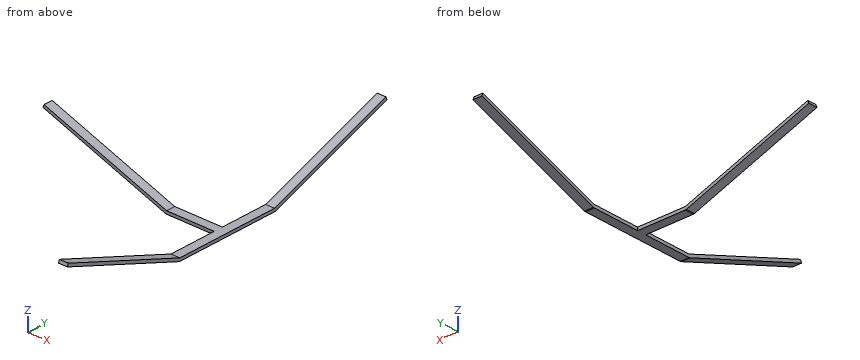
```python
from build123d import *

# Parameters (mm, degrees)
BOSS_EXTRUDE1_DEPTH  = 350
SKETCH2_W            = 150
SKETCH2_H            = 350
BOSS_EXTRUDE2_DEPTH  = 350
BOSS_EXTRUDE3_DEPTH  = 350
BOSS_EXTRUDE4_DEPTH  = 350
SKETCH6_W            = 438.570660024
SKETCH6_H            = 30
CUT_EXTRUDE1_DEPTH   = 10
CUT_EXTRUDE2_DEPTH   = 10
SKETCH8_W            = 30
SKETCH8_H            = 438.570660025
CUT_EXTRUDE3_DEPTH   = 10
SKETCH9_W            = 30
SKETCH9_H            = 438.570660025
CUT_EXTRUDE4_DEPTH   = 10
SKETCH12_W           = 438.570660024
SKETCH12_H           = 30
BOSS_EXTRUDE5_DEPTH  = 10
BOSS_EXTRUDE6_DEPTH  = 10
SKETCH14_W           = 30
SKETCH14_H           = 438.570660025
BOSS_EXTRUDE7_DEPTH  = 10
SKETCH15_W           = 30
SKETCH15_H           = 438.570660025
BOSS_EXTRUDE8_DEPTH  = 10
BOSS_EXTRUDE10_DEPTH = 30
BOSS_EXTRUDE11_DEPTH = 30
BOSS_EXTRUDE12_DEPTH = 30
SKETCH20_W           = 438.570660024
SKETCH20_H           = 160
CUT_EXTRUDE5_DEPTH   = 1000
SKETCH21_W           = 438.570660024
SKETCH21_H           = 160
CUT_EXTRUDE6_DEPTH   = 1000
SKETCH22_W           = 160
SKETCH22_H           = 160
CUT_EXTRUDE7_DEPTH   = 1000
SKETCH23_W           = 160
SKETCH23_H           = 160
CUT_EXTRUDE8_DEPTH   = 1000
SKETCH24_W           = 160
SKETCH24_H           = 438.570660025
CUT_EXTRUDE9_DEPTH   = 1000
SKETCH25_W           = 160
SKETCH25_H           = 438.570660025
CUT_EXTRUDE10_DEPTH  = 1000
SKETCH26_W           = 160
SKETCH26_H           = 350
CUT_EXTRUDE11_DEPTH  = 1000
SKETCH27_W           = 160
SKETCH27_H           = 438.570660025
CUT_EXTRUDE12_DEPTH  = 1000
SKETCH28_W           = 160
SKETCH28_H           = 438.570660025
CUT_EXTRUDE13_DEPTH  = 1000
CUT_EXTRUDE14_DEPTH  = 1000
CUT_EXTRUDE15_DEPTH  = 1000


with BuildPart() as part:
    # Sketch1 → Boss-Extrude1 (new body)
    with BuildSketch(Plane(origin=(0, 0, 0), x_dir=(1, 0, 0), z_dir=(0, 1, 0))):
        Polygon((0, 0), (412.121612918, 0), (412.121612918, 150), align=None)
    extrude(amount=BOSS_EXTRUDE1_DEPTH)

    # Sketch2 → Boss-Extrude2 (add)
    with BuildSketch(Plane(origin=(412.121612918, 0, 0), x_dir=(0, 0, -1), z_dir=(1, 0, 0))):
        with Locations((75, 175)):
            Rectangle(SKETCH2_W, SKETCH2_H)
    extrude(amount=BOSS_EXTRUDE2_DEPTH)

    # Sketch4 → Boss-Extrude3 (add)
    with BuildSketch(Plane(origin=(762.121612918, 0, 0), x_dir=(0, 0, -1), z_dir=(1, 0, 0))):
        Polygon((0, 762.121612918), (150, 350), (0, 350), align=None)
    extrude(amount=-BOSS_EXTRUDE3_DEPTH)

    # Sketch5 → Boss-Extrude4 (add)
    with BuildSketch(Plane(origin=(762.121612918, 0, 0), x_dir=(0, 0, -1), z_dir=(1, 0, 0))):
        Polygon((0, 0), (0, -412.121612918), (150, 0), align=None)
    extrude(amount=-BOSS_EXTRUDE4_DEPTH)

    # Sketch6 → Cut-Extrude1 (cut)
    with BuildSketch(Plane(origin=(0, 0, 0), x_dir=(-0.9396926207859104, 0, 0.34202014332566316), z_dir=(-0.34202014332566316, 0, -0.9396926207859104))):
        with Locations((-219.285330012, 175)):
            Rectangle(SKETCH6_W, SKETCH6_H)
    extrude(amount=-CUT_EXTRUDE1_DEPTH, mode=Mode.SUBTRACT)

    # Sketch7 → Cut-Extrude2 (cut)
    with BuildSketch(Plane(origin=(0, 0, -150), x_dir=(-1, 0, 0), z_dir=(0, 0, -1))):
        Polygon((-412.121612918, 190), (-572.121612918, 190), (-572.121612918, 350), (-602.121612918, 350), (-602.121612918, 190), (-602.121612918, 164.900861359), (-602.121612918, 160), (-602.121612918, 0), (-572.121612918, 0), (-572.121612918, 160), (-412.121612918, 160), align=None)
    extrude(amount=-CUT_EXTRUDE2_DEPTH, mode=Mode.SUBTRACT)

    # Sketch8 → Cut-Extrude3 (cut)
    with BuildSketch(Plane(origin=(0, -48.209070726, -132.453333234), x_dir=(-1, 0, 0), z_dir=(0, -0.34202014332566283, -0.9396926207859106))):
        with Locations((-587.121612918, -167.982308514)):
            Rectangle(SKETCH8_W, SKETCH8_H)
    extrude(amount=-CUT_EXTRUDE3_DEPTH, mode=Mode.SUBTRACT)

    # Sketch9 → Cut-Extrude4 (cut)
    with BuildSketch(Plane(origin=(0, 89.151293181, -244.941164929), x_dir=(-1, 0, 0), z_dir=(0, 0.342020143325663, -0.9396926207859105))):
        with Locations((-587.121612918, 496.874725788)):
            Rectangle(SKETCH9_W, SKETCH9_H)
    extrude(amount=-CUT_EXTRUDE4_DEPTH, mode=Mode.SUBTRACT)

    # Sketch20 → Cut-Extrude5 (cut)
    with BuildSketch(Plane(origin=(0, 0, 0), x_dir=(-0.9396926207859104, 0, 0.34202014332566316), z_dir=(-0.34202014332566316, 0, -0.9396926207859104))):
        with Locations((-219.285330012, 80)):
            Rectangle(SKETCH20_W, SKETCH20_H)
    extrude(amount=-CUT_EXTRUDE5_DEPTH, mode=Mode.SUBTRACT)

    # Sketch21 → Cut-Extrude6 (cut)
    with BuildSketch(Plane(origin=(0, 0, 0), x_dir=(-0.9396926207859104, 0, 0.34202014332566316), z_dir=(-0.34202014332566316, 0, -0.9396926207859104))):
        with Locations((-219.285330012, 270)):
            Rectangle(SKETCH21_W, SKETCH21_H)
    extrude(amount=-CUT_EXTRUDE6_DEPTH, mode=Mode.SUBTRACT)

    # Sketch22 → Cut-Extrude7 (cut)
    with BuildSketch(Plane(origin=(0, 0, -150), x_dir=(-1, 0, 0), z_dir=(0, 0, -1))):
        with Locations((-492.121612918, 270)):
            Rectangle(SKETCH22_W, SKETCH22_H)
    extrude(amount=-CUT_EXTRUDE7_DEPTH, mode=Mode.SUBTRACT)

    # Sketch23 → Cut-Extrude8 (cut)
    with BuildSketch(Plane(origin=(0, 0, -150), x_dir=(-1, 0, 0), z_dir=(0, 0, -1))):
        with Locations((-492.121612918, 80)):
            Rectangle(SKETCH23_W, SKETCH23_H)
    extrude(amount=-CUT_EXTRUDE8_DEPTH, mode=Mode.SUBTRACT)

    # Sketch24 → Cut-Extrude9 (cut)
    with BuildSketch(Plane(origin=(0, -48.209070726, -132.453333234), x_dir=(-1, 0, 0), z_dir=(0, -0.34202014332566283, -0.9396926207859106))):
        with Locations((-492.121612918, -167.982308514)):
            Rectangle(SKETCH24_W, SKETCH24_H)
    extrude(amount=-CUT_EXTRUDE9_DEPTH, mode=Mode.SUBTRACT)

    # Sketch25 → Cut-Extrude10 (cut)
    with BuildSketch(Plane(origin=(0, -48.209070726, -132.453333234), x_dir=(-1, 0, 0), z_dir=(0, -0.34202014332566283, -0.9396926207859106))):
        with Locations((-682.121612918, -167.982308514)):
            Rectangle(SKETCH25_W, SKETCH25_H)
    extrude(amount=-CUT_EXTRUDE10_DEPTH, mode=Mode.SUBTRACT)

    # Sketch26 → Cut-Extrude11 (cut)
    with BuildSketch(Plane(origin=(0, 0, -150), x_dir=(-1, 0, 0), z_dir=(0, 0, -1))):
        with Locations((-682.121612918, 175)):
            Rectangle(SKETCH26_W, SKETCH26_H)
    extrude(amount=-CUT_EXTRUDE11_DEPTH, mode=Mode.SUBTRACT)

    # Sketch27 → Cut-Extrude12 (cut)
    with BuildSketch(Plane(origin=(0, 89.151293181, -244.941164929), x_dir=(-1, 0, 0), z_dir=(0, 0.342020143325663, -0.9396926207859105))):
        with Locations((-682.121612918, 496.874725788)):
            Rectangle(SKETCH27_W, SKETCH27_H)
    extrude(amount=-CUT_EXTRUDE12_DEPTH, mode=Mode.SUBTRACT)

    # Sketch28 → Cut-Extrude13 (cut)
    with BuildSketch(Plane(origin=(0, 89.151293181, -244.941164929), x_dir=(-1, 0, 0), z_dir=(0, 0.342020143325663, -0.9396926207859105))):
        with Locations((-492.121612918, 496.874725788)):
            Rectangle(SKETCH28_W, SKETCH28_H)
    extrude(amount=-CUT_EXTRUDE13_DEPTH, mode=Mode.SUBTRACT)

    # Sketch29 → Cut-Extrude14 (cut)
    with BuildSketch(Plane.XZ.offset(-160)):
        Polygon((572.121612918, 0), (29.238044002, 0), (413.884882725, -140), (572.121612918, -140), align=None)
    extrude(amount=-CUT_EXTRUDE14_DEPTH, mode=Mode.SUBTRACT)

    # Sketch30 → Cut-Extrude15 (cut)
    with BuildSketch(Plane.ZY.offset(-572.121612918)):
        Polygon((-140, 348.236730193), (-140, 1.763269807), (0, -382.883568917), (0, 732.883568917), align=None)
    extrude(amount=-CUT_EXTRUDE15_DEPTH, mode=Mode.SUBTRACT)


with BuildPart() as body_2:
    # Sketch12 → Boss-Extrude5 (new body)
    with BuildSketch(Plane(origin=(0, 0, 0), x_dir=(-0.9396926207859104, 0, 0.34202014332566316), z_dir=(-0.34202014332566316, 0, -0.9396926207859104))):
        with Locations((-219.285330012, 175)):
            Rectangle(SKETCH12_W, SKETCH12_H)
    extrude(amount=BOSS_EXTRUDE5_DEPTH)



with BuildPart() as body_3:
    # Sketch13 → Boss-Extrude6 (new body)
    with BuildSketch(Plane(origin=(0, 0, -150), x_dir=(-1, 0, 0), z_dir=(0, 0, -1))):
        Polygon((-572.121612918, 0), (-572.121612918, 160), (-412.121612918, 160), (-412.121612918, 190), (-572.121612918, 190), (-572.121612918, 350), (-602.121612918, 350), (-602.121612918, 0), align=None)
    extrude(amount=BOSS_EXTRUDE6_DEPTH)



with BuildPart() as body_4:
    # Sketch14 → Boss-Extrude7 (new body)
    with BuildSketch(Plane(origin=(0, -48.209070726, -132.453333234), x_dir=(-1, 0, 0), z_dir=(0, -0.34202014332566283, -0.9396926207859106))):
        with Locations((-587.121612918, -167.982308514)):
            Rectangle(SKETCH14_W, SKETCH14_H)
    extrude(amount=BOSS_EXTRUDE7_DEPTH)



with BuildPart() as body_5:
    # Sketch15 → Boss-Extrude8 (new body)
    with BuildSketch(Plane(origin=(0, 89.151293181, -244.941164929), x_dir=(-1, 0, 0), z_dir=(0, 0.342020143325663, -0.9396926207859105))):
        with Locations((-587.121612918, 496.874725788)):
            Rectangle(SKETCH15_W, SKETCH15_H)
    extrude(amount=BOSS_EXTRUDE8_DEPTH)


with BuildPart() as body_3_1:
    add(body_3.part)

    add(body_5.part)  # Boss-Extrude10 merges body 5
    # Sketch17 → Boss-Extrude10 (add)
    with BuildSketch(Plane(origin=(602.121612918, 0, 0), x_dir=(0, 0, -1), z_dir=(1, 0, 0))):
        Polygon((160, 350), (159.396926208, 353.420201433), (150, 350), align=None)
    extrude(amount=-BOSS_EXTRUDE10_DEPTH)


with BuildPart() as body_4_1:
    add(body_4.part)

    add(body_3_1.part)  # Boss-Extrude11 merges body 3
    # Sketch18 → Boss-Extrude11 (add)
    with BuildSketch(Plane(origin=(602.121612918, 0, 0), x_dir=(0, 0, -1), z_dir=(1, 0, 0))):
        Polygon((159.396926208, -3.420201433), (150, 0), (160, 0), align=None)
    extrude(amount=-BOSS_EXTRUDE11_DEPTH)


with BuildPart() as body_2_1:
    add(body_2.part)

    add(body_4_1.part)  # Boss-Extrude12 merges body 4
    # Sketch19 → Boss-Extrude12 (add)
    with BuildSketch(Plane.XZ.offset(-160)):
        Polygon((408.701411485, -159.396926208), (412.121612918, -150), (412.121612918, -160), align=None)
    extrude(amount=-BOSS_EXTRUDE12_DEPTH)


solid = body_2_1.part
```
The model under review builds one solid part; all positions refer to its coordinate system, in mm. Coordinates: 2 decimals unless noted, no trailing zeros. Order: outer loops, then holes, each group sorted by start corner. A loop starts at its lowest first (then second) coordinate and runs counter-clockwise, first axis right, second up. Notation, with made-up numbers: M 72,-6.75 L 85,-6.75 A24 cw 85,30.25 Z; hole C 59.25,-16.75 d9. An arc over 180 degrees is marked long. One line per question, with ' | ' between items.
(1) Add section A-A, the plane y = 176. Write out the cut boundary in (x, z), then the cut area to 3 significant figures.
Geometry results:
outline: M -3.42,-9.4 L 408.7,-159.4 L 412.12,-160 L 602.12,-160 L 602.12,-150 L 412.12,-150 L 0,0 Z | area: 6,300 mm²
(2) Add section D-D, the plane y = -309.5. Write out the cut boundary in (x, z), then the cut area to 3 significant figures.
Geometry results:
outline: M 572.12,-47.99 L 602.12,-47.99 L 602.12,-37.35 L 572.12,-37.35 Z | area: 319 mm²
(3) Add section C-C, the plane x = 505. Write out the cut boundary in (y, z).
Geometry results:
outline: M 160,-160 L 190,-160 L 190,-150 L 160,-150 Z
(4) Add section B-B, the plane z = -32. Write out the cut boundary in (x, y).
Geometry results:
outline: M 58.68,160 L 87.92,160 L 87.92,190 L 58.68,190 Z; M 572.12,-353.44 L 602.12,-353.44 L 602.12,-324.2 L 572.12,-324.2 Z; M 572.12,674.2 L 602.12,674.2 L 602.12,703.44 L 572.12,703.44 Z
(5) For probe 1 along X at (y, z) = (603.5, -62.5); probe 2 along Y at (x, z) = (554, -151), list the stretches that pass through material, from the lowest coordinate up. Write a range as from..to.
Geometry results:
probe 1: x = 572.12..602.12 | probe 2: y = 160..190
(6) Insertion check: pin 1 (5 mm diameter, centred on y = 472, z = -110.5, fed in from -X). The pin has a flat end and moves straight along its axis. Give the tip position at first contact, or say it passes through.
Geometry results:
pin 1: stops at x = 572.12
